from build123d import *

# Parameters (mm, degrees)
BOSS_EXTRU_1_DEPTH = 2


with BuildPart() as part:
    # Esquisse1 → Boss.-Extru.1 (new body)
    with BuildSketch(Plane(origin=(0, 0, 0), x_dir=(0, 0, -1), z_dir=(1, 0, 0))):
        with BuildLine():
            Line((14.696938457, 3), (39.803847577, 3))
            Line((39.803847577, 3), (45, 0))
            Line((45, 0), (39.803847577, -3))
            Line((39.803847577, -3), (14.696938457, -3))
            ThreePointArc((14.696938457, -3), (-15, 0), (14.696938457, 3))
        make_face()
        with BuildLine():
            Line((-4.663689527, -6.5), (4.663689527, -6.5))
            ThreePointArc((4.663689527, -6.5), (8, 0), (4.663689527, 6.5))
            Line((4.663689527, 6.5), (-4.663689527, 6.5))
            ThreePointArc((-4.663689527, 6.5), (-8, 0), (-4.663689527, -6.5))
        make_face(mode=Mode.SUBTRACT)
    extrude(amount=BOSS_EXTRU_1_DEPTH)


solid = part.part
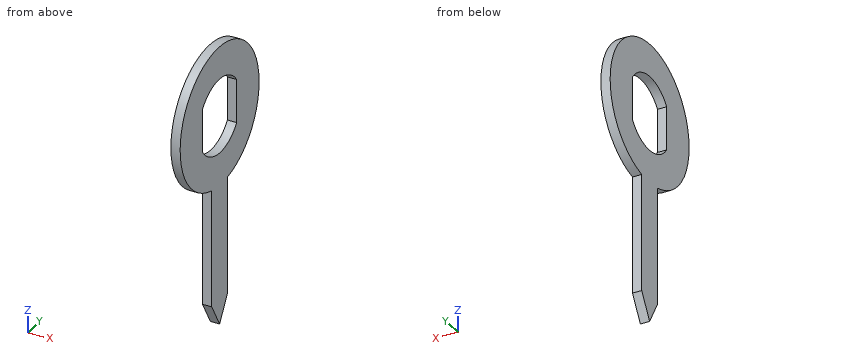
Geometry: final body of the model. Coordinates: model frame, mm. Round coordinates to 2 decimals unless told otherwise and drop trailing zeros. Order: outer loops, then holes, each group sorted by start corner. A loop starts at its lowest first (then second) coordinate and runs counter-clockwise, first axis right, second up. Notation, with made-up numbers: (87, -28.5) -> (108, -28.5) arc R24 ccw to (108, -7.5) -> close; hole circle Ø8 at (-19.5, 83). An arc over 180 degrees is marked (long way). Put each result on its own line as item: value. Start each with the question number.
Q1. Line query: probe 1 along Y at (x, z) = (0.8, -36.5); probe 2 along Z at (x, y) = (1.2, 6); probe 3 along Y at (x, z) = (0.45, -5) (3 decimals). Output: solid intervals per line, ascending.
Q2. Section D-D on z = -15.5. Return the cut outline in (x, y).
Q3. Section A-A on z = 0. Return the cut outline in (x, y), and give its area (3 significant figures).
Q4. Section B-B on x = 0.75. Return the cut outline in (y, z), and give its area (3 significant figures).
Q5. First-contact query: pin 1 (1 mm diameter, centred on x = 1, z = -2.5, fed in from -Y); pin 2 (1 mm diameter, centred on x = 2, y = -6, fed in from +Z). Flat tips, straight axial feed; report the tip coordinate or a pass-through.
Q6. Section C-C on y = -5. Return the cut outline in (x, z) (3 decimals).
Ans:
1. probe 1: y = -3 to 3
1. probe 2: z = -13.75 to -5.29, 5.29 to 13.75
1. probe 3: y = -14.142 to -6.245, 6.245 to 14.142
2. outline: (0, -3) -> (2, -3) -> (2, 3) -> (0, 3) -> close
3. outline: (0, -15) -> (2, -15) -> (2, -6.5) -> (0, -6.5) -> close; (0, 6.5) -> (2, 6.5) -> (2, 15) -> (0, 15) -> close
3. area: 34.0 mm2
4. outline: (-3, -39.8) -> (0, -45) -> (3, -39.8) -> (3, -14.7) arc R15 ccw (long way) to (-3, -14.7) -> close; hole (-6.5, -4.66) arc R8 ccw to (6.5, -4.66) -> (6.5, 4.66) arc R8 ccw to (-6.5, 4.66) -> close
4. area: 690 mm2
5. pin 1: stops at y = -14.87
5. pin 2: stops at z = 13.96
6. outline: (0, -14.142) -> (2, -14.142) -> (2, -6.245) -> (0, -6.245) -> close; (0, 6.245) -> (2, 6.245) -> (2, 14.142) -> (0, 14.142) -> close
